Build history of the part. All positions in model axes, mm. A direction names the side the tool comes from. Round coordinates to 2 decimals unless told otherwise and drop trailing zeros. Order: outer loops, then holes, each group sorted by start corner. A loop starts at its lowest first (then second) coordinate and runs counter-clockwise, first axis right, second up. Notation, with made-up numbers: M -16.5,65.5 L -2.5,65.5 A26 ccw -2.5,86.5 Z; hole C -22.75,-16 d8. An arc over 180 degrees is marked long. One line per item, written item: value. Start each with the question number.
Item 1: Band-saw the part on B-B, the plane x = -9.2. Write the cut outline in (y, z).
Item 2: Band-saw the part on C-C, the plane y = 2. Write the cut outline in (x, z).
Item 3: Band-saw the part on D-D, the plane z = 4.5. Write the cut outline in (x, y), then the cut area to 3 significant figures.
Item 4: Tool access for faces 1 (the flat face through (0, 8, -3.8)), 2 (the flat face through (0, -7, 3.6)), 3 (the flat face through (3.15, 3, 5)): list every direction of +Z, -Z, +X, -X, +Y, -Y with a clear straight run to the whole face (end or side of a thin tool).
Item 5: Two-plate mould, pull along X, no slides. Class faces 4 (the flat face through (8, 0, -6.6)), 5 (the flat face through (0.1, 6.6, -4.4)), 6 (the cylindrical face through (13.33, -14.4, -0.09)): +X half, -X half, draft (parallel to the pull), parting line (faces both ways), or undercut.
Item 6: Pin check, flat tips, straight feed: pin 1 (2 mm diameter, centred on x = 2, y = 5.5, fed in from +Z); pin 2 (0.5 mm diameter, centred on x = 0.5, z = -4, fed in from -Y); pin 3 (0.9 mm diameter, centred on x = 0, y = 6.5, fed in from -Z); pin 4 (4.5 mm diameter, centred on x = -1.5, y = 0, fed in from -Z). Stop position of each tip, or through.
Item 7: Band-saw the part on A-A, the plane z = 0.5. Write the cut outline in (x, y), then the cut area to 3 significant figures.
Item 8: Probe L1, parallel to Y at x = 9.2, z = 3; L2, parallel to X at y = -10.3, z = -3; L3, parallel to Y at x = 0, z = 5. List the from-to ranges inside material, lowest first.
```python
from build123d import *

# Parameters (mm, degrees)
SKETCH2_W               = 27.8
SKETCH2_H               = 13.2
BOSS_EXTRUDE1_DEPTH     = 15
SKETCH7_R               = 1.7
CUT_EXTRUDE1_DEPTH      = 25.340295808
MIRROR2_COPY_1_SKETCH_R = 1.7
MIRROR2_COPY_1_DEPTH    = 25.340295808
SKETCH8_W               = 8.3
SKETCH8_H               = 10.2
CUT_EXTRUDE2_DEPTH      = 21.2
CUT_EXTRUDE5_START      = 1
CUT_EXTRUDE5_DEPTH      = 6.3
SKETCH12_W              = 6.3
SKETCH12_H              = 6.3
CUT_EXTRUDE6_DEPTH      = 23.852789764
FILLET4_R               = 0.5
FILLET3_R               = 2
FILLET5_R               = 0.5
SKETCH13_R              = 1.7
CUT_EXTRUDE7_DEPTH      = 27.195610319


with BuildPart() as part:
    # Sketch2 → Boss-Extrude1 (new, symmetric)
    with BuildSketch(Plane(origin=(0, 0, 0), x_dir=(1, 0, 0), z_dir=(0, 1, 0))):
        Rectangle(SKETCH2_W, SKETCH2_H)
    extrude(amount=BOSS_EXTRUDE1_DEPTH, both=True)

    # Sketch7 → Cut-Extrude1 (cut, through all)
    with BuildSketch(Plane.XY.offset(6.6)):
        with Locations((-9.2, 10.3)):
            Circle(SKETCH7_R)
    cut_extrude1 = extrude(amount=-CUT_EXTRUDE1_DEPTH, mode=Mode.SUBTRACT)

    # Mirror1: Cut-Extrude1 across plane
    add(cut_extrude1.mirror(Plane(origin=(0, 0, 0), x_dir=(0, 0, 1), z_dir=(1, 0, 0))), mode=Mode.SUBTRACT)

    # Mirror2: Cut-Extrude1 across plane
    add(cut_extrude1.mirror(Plane.ZX), mode=Mode.SUBTRACT)

    # Mirror2 copy 1 sketch → Mirror2 copy 1 (cut, through all)
    with BuildSketch(Plane(origin=(0, 0, 6.6), x_dir=(-1, 0, 0), z_dir=(0, 0, 1))):
        with Locations((-9.2, 10.3)):
            Circle(MIRROR2_COPY_1_SKETCH_R)
    extrude(amount=-MIRROR2_COPY_1_DEPTH, mode=Mode.SUBTRACT)

    # Sketch8 → Cut-Extrude2 (cut)
    with BuildSketch(Plane.XZ.offset(15)):
        with Locations((0, -1.5)):
            Rectangle(SKETCH8_W, SKETCH8_H)
    extrude(amount=-CUT_EXTRUDE2_DEPTH, mode=Mode.SUBTRACT)

    # Sketch11 → Cut-Extrude5 (cut)
    with BuildSketch(Plane.ZY.offset(-4.15).offset(CUT_EXTRUDE5_START)):
        Polygon((-11.6, 15), (-4.4, 15), (-4.4, 14.2), (-3.8, 14.2), (-3.8, 13), (-4.4, 13), (-4.4, 12.2), (-3.8, 12.2), (-3.8, 11), (-4.4, 11), (-4.4, 10.2), (-3.8, 10.2), (-3.8, 9), (-4.4, 9), (-4.4, 8.2), (-3.8, 8.2), (-3.8, 7), (-4.4, 7), (-4.4, 6.2), (-11.6, 6.2), align=None)
    extrude(amount=CUT_EXTRUDE5_DEPTH, mode=Mode.SUBTRACT)

    # Sketch12 → Cut-Extrude6 (cut, through all)
    with BuildSketch(Plane(origin=(0, 0, 3.6), x_dir=(-1, 0, 0), z_dir=(0, 0, -1))):
        with Locations((0, 3.05)):
            Rectangle(SKETCH12_W, SKETCH12_H)
    extrude(amount=-CUT_EXTRUDE6_DEPTH, mode=Mode.SUBTRACT)

    # Fillet4
    fillet4_edges = [part.edges().sort_by_distance(p)[0] for p in [
        (-3.15, 6.2, 5.1),
        (-3.15, -0.1, 5.1),
        (3.15, -0.1, 5.1),
        (3.15, 6.2, 5.1),
    ]]
    fillet(fillet4_edges, radius=FILLET4_R)

    # Fillet3
    fillet3_edges = [part.edges().sort_by_distance(p)[0] for p in [
        (-13.9, 15, 0),
        (13.9, 15, 0),
        (-13.9, -15, 0),
        (13.9, -15, 0),
    ]]
    fillet(fillet3_edges, radius=FILLET3_R)

    # Fillet5
    fillet5_edges = [part.edges().sort_by_distance(p)[0] for p in [
        (4.15, -15, -1.5),
        (-4.15, -15, -1.5),
        (-3.15, 6.2, -5.5),
        (3.15, 6.2, -5.5),
        (3.15, 15, -5.5),
        (-3.15, 15, -5.5),
    ]]
    fillet(fillet5_edges, radius=FILLET5_R)

    # Sketch13 → Cut-Extrude7 (cut, through all)
    with BuildSketch(Plane.XZ.offset(-6.2)):
        with Locations(Location((0, 0.5, 0), (0, 0, 270))):
            Circle(SKETCH13_R)
    extrude(amount=-CUT_EXTRUDE7_DEPTH, mode=Mode.SUBTRACT)


solid = part.part
```
Output:
1. outline: M -15,-6.6 L -12,-6.6 L -12,6.6 L -15,6.6 Z; M -8.6,-6.6 L 8.6,-6.6 L 8.6,6.6 L -8.6,6.6 Z; M 12,-6.6 L 15,-6.6 L 15,6.6 L 12,6.6 Z
2. outline: M -13.9,-6.6 L -4.15,-6.6 L -4.15,3.6 L -3.15,3.6 L -3.15,6.6 L -13.9,6.6 Z; M 3.15,3.6 L 4.15,3.6 L 4.15,-6.6 L 13.9,-6.6 L 13.9,6.6 L 3.15,6.6 Z
3. outline: M -13.9,-13 A2 ccw -11.9,-15 L 11.9,-15 A2 ccw 13.9,-13 L 13.9,13 A2 ccw 11.9,15 L -11.9,15 A2 ccw -13.9,13 Z; hole C -9.2,-10.3 d3.4; hole C -9.2,10.3 d3.4; hole M -3.15,0.4 A0.5 ccw -2.65,-0.1 L 2.65,-0.1 A0.5 ccw 3.15,0.4 L 3.15,5.7 A0.5 ccw 2.65,6.2 L -2.65,6.2 A0.5 ccw -3.15,5.7 Z; hole C 9.2,-10.3 d3.4; hole C 9.2,10.3 d3.4
3. area: 755 mm²
4. face 1: -Z
4. face 2: -Z, -Y
4. face 3: +Z, -Z
5. face 4: draft
5. face 5: undercut
5. face 6: +X half
6. pin 1: stops at z = 6.6
6. pin 2: stops at y = 6.2
6. pin 3: stops at z = -4.4
6. pin 4: stops at z = 3.6
7. outline: M -13.9,-13 A2 ccw -11.9,-15 L -4.65,-15 A0.5 ccw -4.15,-14.5 L -4.15,6.2 L -1.7,6.2 L -1.7,15 L -11.9,15 A2 ccw -13.9,13 Z; M 1.7,6.2 L 4.15,6.2 L 4.15,-14.5 A0.5 ccw 4.65,-15 L 11.9,-15 A2 ccw 13.9,-13 L 13.9,13 A2 ccw 11.9,15 L 1.7,15 Z; hole C -9.2,-10.3 d3.4; hole C -9.2,10.3 d3.4; hole C 9.2,-10.3 d3.4; hole C 9.2,10.3 d3.4
7. area: 588 mm²
8. L1: y = -15 to -12, -8.6 to 8.6, 12 to 15
8. L2: x = -13.9 to -10.9, -7.5 to -4.15, 4.15 to 7.5, 10.9 to 13.9
8. L3: y = -15 to -0.1, 6.2 to 15
